```python
from build123d import *

# Parameters (mm, degrees)
MAKERBEAMFIX_DEPTH            = 40
SKETCH4_R                     = 1.25
HOLEFORHARTINGCONNECTOR_DEPTH = 11
FILLET1_R                     = 1
FILLET1_OF_MIRROR1_R          = 1
SKETCH5_W                     = 2.9
SKETCH5_H                     = 30
MAKERBEAMFIXLEFT_DEPTH        = 2
SKETCH6_W                     = 2.9
SKETCH6_H                     = 30
MAKERBEAMFIXRIGHT_DEPTH       = 2


with BuildPart() as part:
    # Sketch1 → MakerBeamFix (new body, symmetric)
    with BuildSketch(Plane.XY):
        Polygon((-5, -15), (-1.45, -15), (-1.45, -17), (1.45, -17), (1.45, -15), (5, -15), (5, 15), (1.45, 15), (1.45, 17), (-1.45, 17), (-1.45, 15), (-5, 15), align=None)
    extrude(amount=MAKERBEAMFIX_DEPTH, both=True)

    # Sketch4 → HoleForHartingConnector (cut, through all)
    with BuildSketch(Plane.ZY.offset(5)):
        with Locations((-31.75, 6.75)):
            Circle(SKETCH4_R)
        with Locations((31.75, 6.75)):
            Circle(SKETCH4_R)
        Polygon((-29.5, 12.5), (29.5, 12.5), (27.5, 1), (-27.5, 1), align=None)
    holeforhartingconnector = extrude(amount=-HOLEFORHARTINGCONNECTOR_DEPTH, mode=Mode.SUBTRACT)

    # Fillet1
    fillet1_edges = [part.edges().sort_by_distance(p)[0] for p in [
        (0, 1, -27.5),
        (0, 12.5, -29.5),
        (0, 12.5, 29.5),
        (0, 1, 27.5),
    ]]
    fillet(fillet1_edges, radius=FILLET1_R)

    # Mirror1: HoleForHartingConnector across plane
    add(holeforhartingconnector.mirror(Plane.ZX), mode=Mode.SUBTRACT)

    # Fillet1 of Mirror1
    fillet1_of_mirror1_edges = [part.edges().sort_by_distance(p)[0] for p in [
        (0, -1, -27.5),
        (0, -12.5, -29.5),
        (0, -12.5, 29.5),
        (0, -1, 27.5),
    ]]
    fillet(fillet1_of_mirror1_edges, radius=FILLET1_OF_MIRROR1_R)

    # Sketch5 → MakerBeamFixLeft (add)
    with BuildSketch(Plane.XY.offset(40)):
        Rectangle(SKETCH5_W, SKETCH5_H)
    extrude(amount=MAKERBEAMFIXLEFT_DEPTH)

    # Sketch6 → MakerBeamFixRight (add)
    with BuildSketch(Plane(origin=(0, 0, -40), x_dir=(-1, 0, 0), z_dir=(0, 0, -1))):
        Rectangle(SKETCH6_W, SKETCH6_H)
    extrude(amount=MAKERBEAMFIXRIGHT_DEPTH)


solid = part.part
```
CAD build for the part. Positions are in the model's coordinates, mm. A direction names the side the tool comes from. Round coordinates to 2 decimals unless told otherwise and drop trailing zeros. Loops run counter-clockwise (first coordinate to the right, second up) from the corner with the lowest first, then second, coordinate; pieces in that order, holes last. Notation, with made-up numbers: (24, 79) - (57, 79) arc R18 cw to (57, 99) - close; hole circle Ø2 at (53.25, -8.5). An arc over 180 degrees is marked (long way). Return JSON: item names as keys, results as strings. Group by question number.
Q1. Band-saw the part on D-D on y = -4.5. Give the cut face in (x, z), plus the area to 3 significant figures.
Q2. Band-saw the part on C-C on x = -3.75. Give the cut face in (y, z).
Q3. Drill centre lines: line 1 along Y through (x, z) = (1, -14.5); line 2 along Y through (x, z) = (-2.25, -5.5); line 3 along Z through (x, y) = (-2.25, -6.75). Where is each one in solid material? Low to high. Write a range as [from, to].
Q4. Tool access for faces 1 (the face through (1.45, -16, 1)), 2 (the face through (-3, 15, 1)), 3 (the face through (0, -12.5, 0)): list every direction of +Z, -Z, +X, -X, +Y, -Y with a clear straight run to the whole face (end or side of a thin tool).
Q5. Flat gauge pins, fed straight in: pin 1 Ø2 at (x, z) = (0, -41.5) entering from +Y; pin 2 Ø4 at (x, y) = (-3.5, 2.5) entering from +Z; pin 3 Ø0.6 at (x, y) = (-0.5, -15.5) entering from -Z. Where does each tip first touch, or does it go through?
Q6. Two-plate mould, pull along Y, no slides. Class faces 4 (the face through (1.45, 0, 41)), 5 (the face through (0, 15, -41)), 6 (the face through (-0.07, -5.641, 32.327)), 7 (the face through (0, -15, 41)): +Y half, -Y half, draft (parallel to the pull), parting line (faces both ways), or undercut.
Q7. Band-saw the part on A-A on z = 18.5. Give the cut face in (x, y).
Q8. Band-saw the part on B-B on y = 6.75. Give the cut face in (x, z).
Solutions:
{
 "1": {"outline": "(-5, -40) - (-1.45, -40) - (-1.45, -42) - (1.45, -42) - (1.45, -40) - (5, -40) - (5, -28.11) - (-5, -28.11) - close; (-5, 28.11) - (5, 28.11) - (5, 40) - (1.45, 40) - (1.45, 42) - (-1.45, 42) - (-1.45, 40) - (-5, 40) - close", "area": "249 mm^2"},
 "2": {"outline": "(-15, -40) - (15, -40) - (15, 40) - (-15, 40) - close; hole (-12.5, -28.31) arc R1 ccw to (-11.33, -29.3) - (-1.83, -27.64) arc R1 ccw to (-1, -26.66) - (-1, 26.66) arc R1 ccw to (-1.83, 27.64) - (-11.33, 29.3) arc R1 ccw to (-12.5, 28.31) - close; hole circle Ø2.5 at (-6.75, -31.75); hole circle Ø2.5 at (-6.75, 31.75); hole (1, -26.66) arc R1 ccw to (1.83, -27.64) - (11.33, -29.3) arc R1 ccw to (12.5, -28.31) - (12.5, 28.31) arc R1 ccw to (11.33, 29.3) - (1.83, 27.64) arc R1 ccw to (1, 26.66) - close; hole circle Ø2.5 at (6.75, -31.75); hole circle Ø2.5 at (6.75, 31.75)"},
 "3": {"line 1": "y = [-17, -12.5], [-1, 1], [12.5, 17]", "line 2": "y = [-15, -12.5], [-1, 1], [12.5, 15]", "line 3": "z = [-40, -33], [-30.5, -28.5], [28.5, 30.5], [33, 40]"},
 "4": {"face 1": "+Z, -Z, +X, -Y", "face 2": "+Z, -Z, -X, +Y", "face 3": "+X, -X"},
 "5": {"pin 1": "stops at y = 15", "pin 2": "stops at z = 40", "pin 3": "stops at z = -40"},
 "6": {"face 4": "draft", "face 5": "+Y half", "face 6": "undercut", "face 7": "-Y half"},
 "7": {"outline": "(-5, -15) - (-1.45, -15) - (-1.45, -17) - (1.45, -17) - (1.45, -15) - (5, -15) - (5, -12.5) - (-5, -12.5) - close; (-5, -1) - (5, -1) - (5, 1) - (-5, 1) - close; (-5, 12.5) - (5, 12.5) - (5, 15) - (1.45, 15) - (1.45, 17) - (-1.45, 17) - (-1.45, 15) - (-5, 15) - close"},
 "8": {"outline": "(-5, -40) - (-1.45, -40) - (-1.45, -42) - (1.45, -42) - (1.45, -40) - (5, -40) - (5, -33) - (-5, -33) - close; (-5, -30.5) - (5, -30.5) - (5, -28.5) - (-5, -28.5) - close; (-5, 28.5) - (5, 28.5) - (5, 30.5) - (-5, 30.5) - close; (-5, 33) - (5, 33) - (5, 40) - (1.45, 40) - (1.45, 42) - (-1.45, 42) - (-1.45, 40) - (-5, 40) - close"}
}
